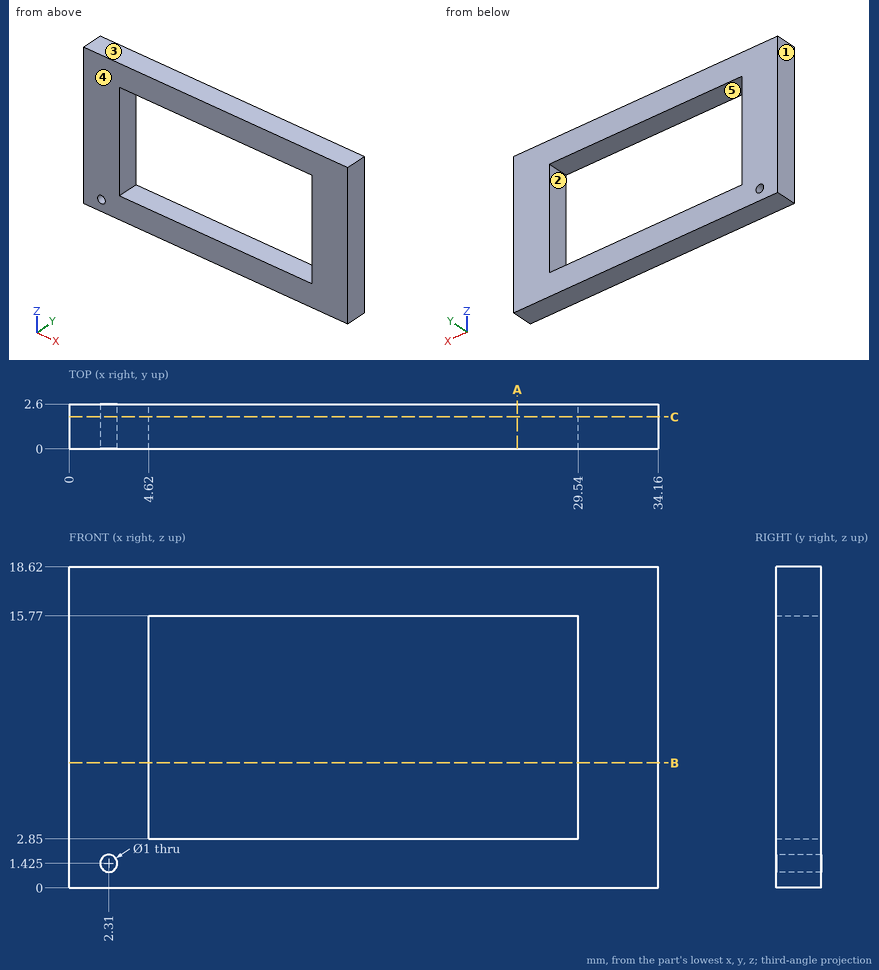
Source: three-view drawing plus pictorial views. Frame: mm from the lowest corner of the part. A direction names the side the tool comes from. Give positions to 0.01 mm unless a question says otherwise; leave off trailing zeros. Loops run counter-clockwise (first coordinate to the right, second up) from the corner with the lowest first, then second, coordinate; pieces in that order, holes last. Notation, with made-up numbers: M 53,-31 L 104,-31 A27 cw 104,6 Z; hole C -26.75,9.5 d8. An arc over 180 degrees is marked long. Put each result on its own line as item: value.
Q1. Section C-C (y = 1.85). Return the cut outline in (x, z) (3 decimals), and give its area (3 significant figures).
Response values:
outline: M 0,0 L 34.16,0 L 34.16,18.62 L 0,18.62 Z; hole C 2.31,1.425 d1; hole M 4.62,2.85 L 29.54,2.85 L 29.54,15.77 L 4.62,15.77 Z
area: 313 mm²
Q2. Mould query, pull axis Z, two halves, no side actions, for the marked faces 3, 4 and 5. Classes: released by +Z, released by -Z, zero draft, split by the parting line, or undercut.
Response values:
face 3: released by +Z
face 4: zero draft
face 5: undercut
Q3. Section B-B (z = 7.25). Return the cut outline in (x, y), and give its area (3 significant figures).
Response values:
outline: M 0,0 L 4.62,0 L 4.62,2.6 L 0,2.6 Z; M 29.54,0 L 34.16,0 L 34.16,2.6 L 29.54,2.6 Z
area: 24.0 mm²
Q4. Line query: probe 1 along X at (y, z) = (1.6, 12); probe 2 along Z at (x, y) = (18, 0.9); probe 3 along Z at (x, y) = (2.31, 1.25) (3 decimals). Output: solid intervals per line, ascending. Write a range as [from, to].
Response values:
probe 1: x = [0, 4.62], [29.54, 34.16]
probe 2: z = [0, 2.85], [15.77, 18.62]
probe 3: z = [0, 0.925], [1.925, 18.62]
Q5. Reachability of the marked faces 1 and 2 from +Z, -Z, +X, -X, +Y, -Y: full face, straight path, thin tool, end or side. Return the list, or none.
Response values:
face 1: +Z, -Z, -X, +Y, -Y
face 2: +Y, -Y
Q6. Section A-A (x = 26). Return the cut outline in (y, z).
Response values:
outline: M 0,0 L 2.6,0 L 2.6,2.85 L 0,2.85 Z; M 0,15.77 L 2.6,15.77 L 2.6,18.62 L 0,18.62 Z
Q7. Pin query (flat end, axial travel): P1, Ø2, axis at x = 22, z = 14, coming from the +Y side. Return the tip coordinate at first contact, or that it passes through.
Response values:
P1: passes through
